Model file for the job. Use its own axes, mm. Face numbers are marked on the shaded views. A direction names the side the tool comes from. Coordinates: 2 decimals unless noted, no trailing zeros. Write each loop counter-clockwise with the first axis right and the second up, starting at its lowest first coordinate (ties: lowest second). Pieces come first, ordered by that corner, then holes. Notation, with made-up numbers: M 32,-32 L 40,-32 A20 ccw 40,-4 Z; hole C 6,-21.5 d3. An arc over 180 degrees is marked long. One line per question, with ' | ' between items. Start each with the question number.
(1) Cut at D-D (x = 15). Write the cut outline in (y, z), plus the area to 3 significant figures.
(2) Cut at A-A (z = 25.4). Write the cut outline in (x, y).
(3) Cut at B-B (y = -12.7). Write the cut outline in (x, z), plus the area to 3 significant figures.
(4) Cut at C-C (x = -8.5). Write the cut outline in (y, z).
(5) Flat gauge pins, fed straight in: pin 1 Ø5 at (x, y) = (19.5, -22.5) entering from -Z; pin 2 Ø6.5 at (x, z) = (17, 33) entering from +Y; pin 3 Ø5 at (y, z) = (13.5, -27.5) entering from -X; pin 4 Ø4 at (y, z) = (6, -26.5) entering from +X. Where does each tip first touch, or does it go through?
(6) Two-plate mould, pull along Z, no slides. Class the marked faces 4, 5 and 6: +Z half, -Z half, draft (parallel to the pull), parting line (faces both ways), or undercut.
(7) Tool access for the marked faces 1, 2 and 3: list every direction of +Z, -Z, +X, -X, +Y, -Y with a clear straight run to the whole face (end or side of a thin tool).
(8) Wall check: probe 1 along Y at (x, z) = (-2.75, 25.4); probe 2 along Y at (x, z) = (0, -20); probe 3 along X at (y, z) = (-12.7, 19). Give the ranges that are in metal, low to high.
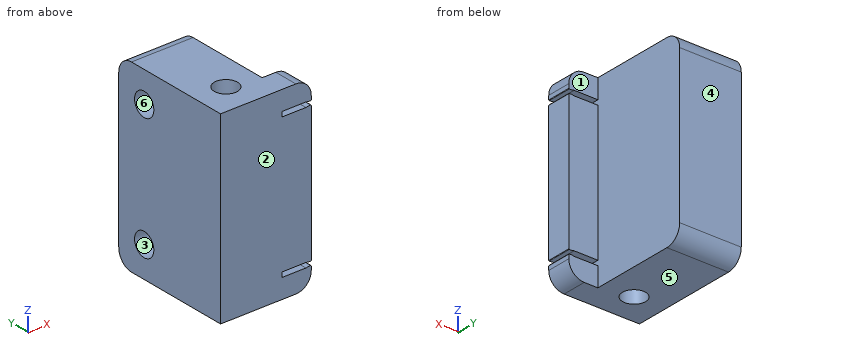
from build123d import *

# Parameters (mm, degrees)
SKETCH1_W           = 25.4
SKETCH1_H           = 50.8
SKETCH1_R           = 4.8006
BOSS_EXTRUDE1_DEPTH = 38.1
SKETCH2_R           = 4.8006
CUT_EXTRUDE1_DEPTH  = 48.519048812
SKETCH3_W           = 12
SKETCH3_H           = 76.2
BOSS_EXTRUDE2_DEPTH = 10
CUT_EXTRUDE2_DEPTH  = 53.027492732
FILLET1_R           = 6.35


with BuildPart() as part:
    # Sketch1 → Boss-Extrude1 (new, symmetric)
    with BuildSketch(Plane.XY):
        Rectangle(SKETCH1_W, SKETCH1_H)
        with Locations(Location((0, -12.7, 0), (0, 0, 180))):
            Circle(SKETCH1_R, mode=Mode.SUBTRACT)
    extrude(amount=BOSS_EXTRUDE1_DEPTH, both=True)

    # Sketch2 → Cut-Extrude1 (cut, through all)
    with BuildSketch(Plane(origin=(0, 0, 0), x_dir=(0, 0, -1), z_dir=(1, 0, 0))):
        with Locations((-25.4, 12.7)):
            Circle(SKETCH2_R)
        with Locations(Location((25.4, 12.7, 0), (0, 0, 180))):
            Circle(SKETCH2_R)
    extrude(amount=-CUT_EXTRUDE1_DEPTH, mode=Mode.SUBTRACT)

    # Sketch3 → Boss-Extrude2 (add)
    with BuildSketch(Plane.XZ.offset(25.4)):
        with Locations((18.7, 0)):
            Rectangle(SKETCH3_W, SKETCH3_H)
    extrude(amount=-BOSS_EXTRUDE2_DEPTH)

    # Sketch4 → Cut-Extrude2 (cut, through all)
    with BuildSketch(Plane(origin=(0, 0, 0), x_dir=(1, 0, 0), z_dir=(0, 1, 0))):
        with BuildLine():
            Line((24.7, 30.1), (24.7, 28.1))
            ThreePointArc((24.7, 28.1), (24.641421356, 28.241421356), (24.5, 28.3))
            ThreePointArc((24.5, 28.3), (23.495012438, 28.249875621), (22.5, 28.1))
            Line((22.5, 28.1), (12.7, 28.1))
            Line((12.7, 28.1), (12.7, 30.1))
            Line((12.7, 30.1), (22.5, 30.1))
            ThreePointArc((22.5, 30.1), (23.495012438, 29.950124379), (24.5, 29.9))
            ThreePointArc((24.5, 29.9), (24.641421356, 29.958578644), (24.7, 30.1))
        make_face()
        with BuildLine():
            Line((24.7, -30.1), (24.7, -28.1))
            ThreePointArc((24.7, -28.1), (24.641421356, -28.241421356), (24.5, -28.3))
            ThreePointArc((24.5, -28.3), (23.495012438, -28.249875621), (22.5, -28.1))
            Line((22.5, -28.1), (12.7, -28.1))
            Line((12.7, -28.1), (12.7, -30.1))
            Line((12.7, -30.1), (22.5, -30.1))
            ThreePointArc((22.5, -30.1), (23.495012438, -29.950124379), (24.5, -29.9))
            ThreePointArc((24.5, -29.9), (24.641421356, -29.958578644), (24.7, -30.1))
        make_face()
    extrude(amount=-CUT_EXTRUDE2_DEPTH, mode=Mode.SUBTRACT)

    # Fillet1
    fillet1_edges = [part.edges().sort_by_distance(p)[0] for p in [
        (24.7, -20.4, 38.1),
        (24.7, -20.4, -38.1),
        (0, 25.4, -38.1),
        (0, 25.4, 38.1),
    ]]
    fillet(fillet1_edges, radius=FILLET1_R)


solid = part.part
Filled in:
1) outline: M -25.4,-38.1 L -15.4,-38.1 L -15.4,-30.1 L -25.4,-30.1 Z; M -25.4,-28.1 L -15.4,-28.1 L -15.4,28.1 L -25.4,28.1 Z; M -25.4,30.1 L -15.4,30.1 L -15.4,38.1 L -25.4,38.1 Z | area: 722 mm²
2) outline: M -12.7,-25.4 L 24.7,-25.4 L 24.7,-15.4 L 12.7,-15.4 L 12.7,25.4 L -12.7,25.4 L -12.7,17.5 L 0,17.5 L 0,7.9 L -12.7,7.9 Z; hole C 0,-12.7 d9.6
3) outline: M -12.7,-38.1 L -4.8,-38.1 L -4.8,38.1 L -12.7,38.1 Z; M 4.8,-38.1 L 12.7,-38.1 L 12.7,38.1 L 4.8,38.1 Z | area: 1,200 mm²
4) outline: M -25.4,-38.1 L 19.05,-38.1 A6.35 ccw 25.4,-31.75 L 25.4,31.75 A6.35 ccw 19.05,38.1 L -25.4,38.1 Z; hole C 12.7,-25.4 d9.6; hole C 12.7,25.4 d9.6
5) pin 1: z = -38.1 | pin 2: y = -15.4 | pin 3: x = 0 | pin 4: x = 12.7
6) face 4: draft | face 5: -Z half | face 6: undercut
7) face 1: +Z, -Z, +X, +Y | face 2: +Z, -Z, +X, -X, -Y | face 3: -X
8) probe 1: -25.4 to -16.63, -8.77 to 7.9, 17.5 to 25.4 | probe 2: -25.4 to -17.5, -7.9 to 25.4 | probe 3: -12.7 to -4.8, 4.8 to 12.7
